from build123d import *

# Parameters (mm, degrees)
F0_R            = 238.1
F1_DEPTH        = 60.15
F1_DEPTH_BACK   = 60.15
F3_D            = 130
F5_D            = 25
F5_CBORE_D      = 58
F5_CBORE_DEPTH  = 40
F5_COPIES_COUNT = 3
F6_R            = 29
F7_DEPTH        = 40
F7_COPIES_COUNT = 3


# Not quite as in the source:
# - a pattern or mirror of a feature is missing from the dataset's text; its kind, count and spacing are read off the source's solid
# - a feature names something its author has since deleted; it is built from what else it names


with BuildPart() as f1:
    # F0 (on Front) → F1 (new body, two sides)
    with BuildSketch(Plane.XZ) as f1_sk:
        Circle(F0_R)
    extrude(amount=F1_DEPTH)
    extrude(f1_sk.sketch, amount=-F1_DEPTH_BACK)

    # F3 (through all)
    with Locations(Plane.XZ.offset(60.15)):
        with Locations((0, 0)):
            Hole(F3_D / 2)

    # F5 (through all)
    with Locations(Plane.XZ.offset(60.15)):
        with Locations((0, -120)):
            f5 = CounterBoreHole(F5_D / 2, F5_CBORE_D / 2, F5_CBORE_DEPTH)

    # F5_copies: F5 ×3 about axis
    f5_copies_axis = Axis((0, 0, 0), (0, 1, 0))
    for i in range(1, F5_COPIES_COUNT):
        add(f5.rotate(f5_copies_axis, i * 360 / F5_COPIES_COUNT), mode=Mode.SUBTRACT)

    # F6 (on face) → F7 (cut)
    with BuildSketch(Plane(origin=(0, 60.15, 0), x_dir=(-1, 0, 0), z_dir=(0, 1, 0))):
        with Locations((0, 120)):
            Circle(F6_R)
    f7 = extrude(amount=-F7_DEPTH, mode=Mode.SUBTRACT)

    # F7_copies: F7 ×3 about axis
    f7_copies_axis = Axis((0, 0, 0), (0, 1, 0))
    for i in range(1, F7_COPIES_COUNT):
        add(f7.rotate(f7_copies_axis, i * 360 / F7_COPIES_COUNT), mode=Mode.SUBTRACT)

    # F8 (on Right) → F9 (revolve, cut)
    with BuildSketch(Plane.YZ):
        with BuildLine():
            Line((-36.55, 205.69), (-11.8, 205.69))
            Line((-11.8, 205.69), (-11.8, 230.69))
            ThreePointArc((-11.8, 230.69), (-11.4200720085, 234.4705976243), (-10.295482274, 238.1))
            Line((-10.295482274, 238.1), (10.295482274, 238.1))
            ThreePointArc((10.295482274, 238.1), (11.4200720085, 234.4705976243), (11.8, 230.69))
            Line((11.8, 230.69), (11.8, 205.69))
            Line((11.8, 205.69), (36.55, 205.69))
            Line((36.55, 205.69), (36.55, 230.69))
            ThreePointArc((36.55, 230.69), (36.9299279915, 234.4705976243), (38.054517726, 238.1))
            Line((38.054517726, 238.1), (58.645482274, 238.1))
            ThreePointArc((58.645482274, 238.1), (59.7700720085, 234.4705976243), (60.15, 230.69))
            Line((60.15, 230.69), (60.15, 223.28))
            Line((60.15, 223.28), (86.0586377919, 223.28))
            Line((86.0586377919, 223.28), (86.0586377919, 283.6410403252))
            Line((86.0586377919, 283.6410403252), (-71.6444390953, 283.6410403252))
            Line((-71.6444390953, 283.6410403252), (-71.6444390953, 224.8791903257))
            Line((-71.6444390953, 224.8791903257), (-60.15, 224.8791903257))
            Line((-60.15, 224.8791903257), (-60.15, 230.69))
            ThreePointArc((-60.15, 230.69), (-59.7700720085, 234.4705976243), (-58.645482274, 238.1))
            Line((-58.645482274, 238.1), (-38.054517726, 238.1))
            ThreePointArc((-38.054517726, 238.1), (-36.9299279915, 234.4705976243), (-36.55, 230.69))
            Line((-36.55, 230.69), (-36.55, 205.69))
        make_face()
    revolve(axis=Axis((0, 0, 0), (0, 1, 0)), mode=Mode.SUBTRACT)


solid = f1.part
The listing builds one solid part. Answer for the finished solid, in the listing's coordinates (mm). A direction names the side the tool comes from. Give positions to 0.01 mm unless a question says otherwise; leave off trailing zeros. Loops run counter-clockwise (first coordinate to the right, second up) from the corner with the lowest first, then second, coordinate; pieces in that order, holes last. Notation, with made-up numbers: M 84,78 L 119,78 A15 ccw 119,83 Z; hole C -15.5,5 d8. An arc over 180 degrees is marked long. Answer as CSV lines item,"result".
Item 1: Straight lines are drawn through the part: line 1 along Y through (x, z) = (-184.5, -136); line 2 along Z through (x, y) = (0, 41); line 3 along Z through (x, y) = (-25, 43.5). For each, find the intervals that lie inside material, in ascending order. Write a range as [from, to].
Values follow:
line 1,"y = [-60.15, -36.55], [-11.8, 11.8], [36.55, 60.15]"
line 2,"z = [-238.1, -132.5], [-107.5, -65], [65, 91], [149, 238.1]"
line 3,"z = [-236.78, -60], [60, 105.3], [134.7, 236.78]"
Item 2: Given pin 1 Ø10 at (x, y) = (148, -40) entering from -Z; pin 2 Ø2 at (y, z) = (-8.5, 81.5) entering from -X; pin 3 Ø4 at (y, z) = (-0.5, 128.5) entering from -X, each flat-ended and moving along its own axis, determine where each tip first touches the part or whether it passes through.
Values follow:
pin 1,"stops at z = -190.37"
pin 2,"stops at x = -224.08"
pin 3,"stops at x = -201.72"
Item 3: The mould has two halves that part along Y. Classify faces 6 (the flat face through (1, -11.8, 206)), 7 (the flat face through (1, -36.55, -206)), 8 (the flat face through (48, -60.15, -48)), 9 (the cylindrical face through (6.29, 40.43, 91.69)): released by +Y, released by -Y, zero draft, split by the parting line, or undercut.
Values follow:
face 6,"undercut"
face 7,"undercut"
face 8,"released by -Y"
face 9,"zero draft"
Item 4: Which of the six approach directions +Z, -Z, +X, -X, +Y, -Y give full straight-line access (tool end or side, diameter ignored) to faces 1 (the cylindrical face through (227.105, -0.144, 71.519)), 2 (the flat face through (-48, 60.15, 48)), 3 (the flat face through (104, 20.15, -61)), 4 (the cylindrical face through (130.71, -40.43, 48.89)), 5 (the flat face through (1, 11.8, -206))?
Values follow:
face 1,"+Y, -Y"
face 2,"+Z, -Z, +X, -X, +Y"
face 3,"+Y"
face 4,"-Y"
face 5,"none"
Item 5: The part is cut by section B-B (x = 0). Give the number of separate pieces and of enclosed holes in the cut face, and give its area (3 significant figures).
Values follow:
separate pieces,"3"
enclosed holes,"0"
area,"31,700 mm^2"
Item 6: The part is cut by section A-A (y = -31). Give the vertices of the cut face in (x, z).
Values follow:
outline,"C 0,0 d411.38; hole C -103.92,60 d58; hole C 0,0 d130; hole C 0,-120 d58; hole C 103.92,60 d58"
